Here's the drawing with two shaded views (mm, measured from the low corner). I have some questions. Give positions to 0.01 mm unless a question says otherwise; leave off trailing zeros. Write each loop counter-clockwise with the first axis right and the second up, starting at its lowest first coordinate (ties: lowest second). Pieces come first, ordered by that corner, then holes. Notation, with made-up numbers: M 9,9.25 L 24,9.25 A31 ccw 24,36.25 Z; hole C 66.25,31.5 d4. An arc over 180 degrees is marked long. Use one line per item in the form item = value. Start each with the question number.
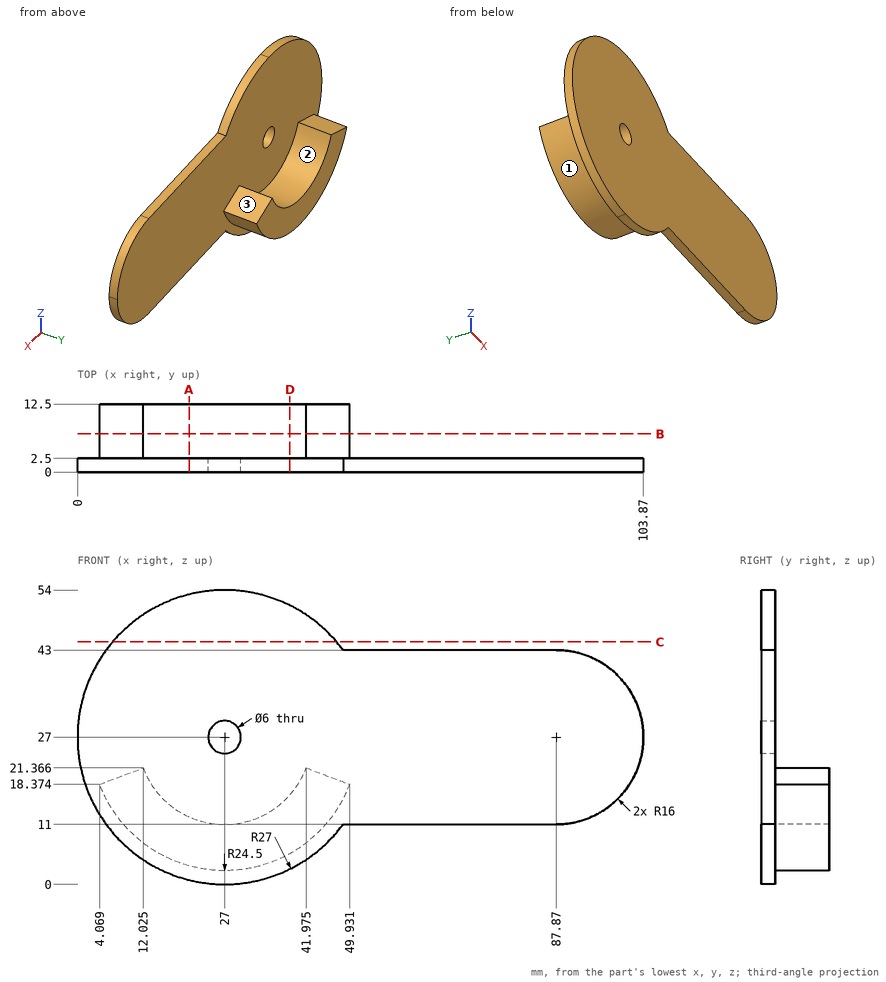
1) Suppose I cut it at A-A, the plane x = 20.5. List the corners of the cut face in (y, z) for me, and give its area (3 significant figures).
2) Will these pins go through, and if not, where does the flat tip stop? P1, Ø2, axis at x = 63.5, y = 1, coming from the -Z side; P2, Ø12, axis at x = 83, z = 9, coming from the +Y side; P3, Ø1, axis at y = 7.5, z = 6, coming from the -X side (1 decimal).
3) Thinking about a two-plate mould opening in X: for the marked faces 1, 2 and 3, which applies, released by +X, released by -X, zero draft, split by the parting line, or undercut?
4) Suppose I cut it at D-D, the plane x = 39. List the corners of the cut face in (y, z) for me, and give its area (3 significant figures).
5) Please list where these lines run through material, in increasing order: line 1 (Y direction, x = 95, z = 19); line 2 (X direction, y = 7.5, z = 13) (1 decimal); line 3 (Z direction, x = 28, y = 3.75).
6) Suppose I cut it at B-B, the plane y = 7. List the corners of the cut face in (x, z) for me (1 decimal), and give its area (3 significant figures).
7) Suppose I cut it at C-C, the plane z = 44.5. List the corners of the cut face in (x, y) for me, and give its area (3 significant figures).
Checks:
q1.outline = M 0,0.79 L 2.5,0.79 L 2.5,3.38 L 12.5,3.38 L 12.5,12.38 L 2.5,12.38 L 2.5,53.21 L 0,53.21 Z
q1.area = 221 mm^2
q2.P1 = 11
q2.P2 = 2.5
q2.P3 = 13.6
q3.face_1 = split by the parting line
q3.face_2 = undercut
q3.face_3 = released by +X
q4.outline = M 0,2.81 L 2.5,2.81 L 2.5,5.64 L 12.5,5.64 L 12.5,16.42 L 2.5,16.42 L 2.5,51.19 L 0,51.19 Z
q4.area = 229 mm^2
q5.line_1 = 0 to 2.5
q5.line_2 = 6.9 to 19.3, 34.7 to 47.1
q5.line_3 = 2.52 to 11.03
q6.outline = M 4.1,18.4 A24.5 ccw 49.9,18.4 L 42,21.4 A16 cw 12,21.4 Z
q6.area = 417 mm^2
q7.outline = M 6.44,0 L 47.56,0 L 47.56,2.5 L 6.44,2.5 Z
q7.area = 103 mm^2
